from build123d import *

# Parameters (mm, degrees)
CORTAR_EXTRUIR1_START                       = 1
CROQUIS2_R                                  = 7.435198433
CORTAR_EXTRUIR1_DEPTH                       = 7
CHAFL_N1_SIZE                               = 0.1
DI_METRO_DE_TALADRO_1_0_1_1_D               = 1
DI_METRO_DE_TALADRO_1_0_1_1_DEPTH           = 0.2
DI_METRO_DE_TALADRO_1_0_1_1_TIP             = 0.30043031
DI_METRO_DE_TALADRO_1_0_1_1_ON_FACE_2_D     = 1
DI_METRO_DE_TALADRO_1_0_1_1_ON_FACE_2_DEPTH = 0.2
DI_METRO_DE_TALADRO_1_0_1_1_ON_FACE_2_TIP   = 0.30043031
DI_METRO_DE_TALADRO_1_0_1_1_ON_FACE_3_D     = 1
DI_METRO_DE_TALADRO_1_0_1_1_ON_FACE_3_DEPTH = 0.2
DI_METRO_DE_TALADRO_1_0_1_1_ON_FACE_3_TIP   = 0.30043031
DI_METRO_DE_TALADRO_1_0_1_1_ON_FACE_4_D     = 1
DI_METRO_DE_TALADRO_1_0_1_1_ON_FACE_4_DEPTH = 0.2
DI_METRO_DE_TALADRO_1_0_1_1_ON_FACE_4_TIP   = 0.30043031
DI_METRO_DE_TALADRO_1_0_1_1_ON_FACE_5_D     = 1
DI_METRO_DE_TALADRO_1_0_1_1_ON_FACE_5_DEPTH = 0.2
DI_METRO_DE_TALADRO_1_0_1_1_ON_FACE_5_TIP   = 0.30043031
DI_METRO_DE_TALADRO_1_0_1_1_ON_FACE_6_D     = 1
DI_METRO_DE_TALADRO_1_0_1_1_ON_FACE_6_DEPTH = 0.2
DI_METRO_DE_TALADRO_1_0_1_1_ON_FACE_6_TIP   = 0.30043031


with BuildPart() as part:
    # Croquis1 → Revolución1 (revolve)
    with BuildSketch(Plane.XY):
        with BuildLine():
            Line((0.5, 0), (0.575, 0))
            ThreePointArc((0.575, 0), (0.759699445, 0.045195667), (0.902660818, 0.170569425))
            Line((0.902660818, 0.170569425), (3.934160742, 4.5))
            Line((3.934160742, 4.5), (6.64058638, 4.5))
            Line((6.64058638, 4.5), (6.64058638, 8.36517638))
            Line((6.64058638, 8.36517638), (7.435198433, 9.5))
            Line((7.435198433, 9.5), (3, 9.5))
            Line((3, 9.5), (3, 19))
            Line((3, 19), (1.6, 19))
            Line((1.6, 19), (1.6, 3.570962807))
            Line((1.6, 3.570962807), (0.5, 2))
            Line((0.5, 2), (0.5, 0))
        make_face()
    revolve(axis=Axis((0, 0, 0), (0, 1, 0)))

    # Croquis2 → Cortar-Extruir1 (cut)
    with BuildSketch(Plane(origin=(0, 9.5, 0), x_dir=(1, 0, 0), z_dir=(0, 1, 0)).offset(CORTAR_EXTRUIR1_START)):
        Circle(CROQUIS2_R)
        Polygon((2.309401077, 4), (-2.309401077, 4), (-4.618802154, 0), (-2.309401077, -4), (2.309401077, -4), (4.618802154, 0), align=None, mode=Mode.SUBTRACT)
    extrude(amount=-CORTAR_EXTRUIR1_DEPTH, mode=Mode.SUBTRACT)

    # Chaflán1
    chafl_n1_edges = [part.edges().sort_by_distance(p)[0] for p in [
        (-1.6, 19, 0),
    ]]
    chamfer(chafl_n1_edges, length=CHAFL_N1_SIZE)

    # Diámetro de taladro Ø1.0 (1)1
    with Locations(Plane(origin=(0, 7, 4), x_dir=(1, 0, 0), z_dir=(0, 0, 1))):
        with Locations((0, 0)):
            Hole(DI_METRO_DE_TALADRO_1_0_1_1_D / 2, depth=DI_METRO_DE_TALADRO_1_0_1_1_DEPTH)
            with Locations((0, 0, -(DI_METRO_DE_TALADRO_1_0_1_1_DEPTH + DI_METRO_DE_TALADRO_1_0_1_1_TIP / 2))):  # 118° drill point
                Cone(0, DI_METRO_DE_TALADRO_1_0_1_1_D / 2, DI_METRO_DE_TALADRO_1_0_1_1_TIP, mode=Mode.SUBTRACT)

    # Diámetro de taladro Ø1.0 (1)1 on face 2
    with Locations(Plane(origin=(3.464101615, 7, 2), x_dir=(-0.500000175, 0, 0.866025303), z_dir=(0.866025303, 0, 0.500000175))):
        with Locations((0, 0)):
            Hole(DI_METRO_DE_TALADRO_1_0_1_1_ON_FACE_2_D / 2, depth=DI_METRO_DE_TALADRO_1_0_1_1_ON_FACE_2_DEPTH)
            with Locations((0, 0, -(DI_METRO_DE_TALADRO_1_0_1_1_ON_FACE_2_DEPTH + DI_METRO_DE_TALADRO_1_0_1_1_ON_FACE_2_TIP / 2))):  # 118° drill point
                Cone(0, DI_METRO_DE_TALADRO_1_0_1_1_ON_FACE_2_D / 2, DI_METRO_DE_TALADRO_1_0_1_1_ON_FACE_2_TIP, mode=Mode.SUBTRACT)

    # Diámetro de taladro Ø1.0 (1)1 on face 3
    with Locations(Plane(origin=(3.464101615, 7, -2), x_dir=(0.500000175, 0, 0.866025303), z_dir=(0.866025303, 0, -0.500000175))):
        with Locations((0, 0)):
            Hole(DI_METRO_DE_TALADRO_1_0_1_1_ON_FACE_3_D / 2, depth=DI_METRO_DE_TALADRO_1_0_1_1_ON_FACE_3_DEPTH)
            with Locations((0, 0, -(DI_METRO_DE_TALADRO_1_0_1_1_ON_FACE_3_DEPTH + DI_METRO_DE_TALADRO_1_0_1_1_ON_FACE_3_TIP / 2))):  # 118° drill point
                Cone(0, DI_METRO_DE_TALADRO_1_0_1_1_ON_FACE_3_D / 2, DI_METRO_DE_TALADRO_1_0_1_1_ON_FACE_3_TIP, mode=Mode.SUBTRACT)

    # Diámetro de taladro Ø1.0 (1)1 on face 4
    with Locations(Plane(origin=(0, 7, -4), x_dir=(-1, 0, 0), z_dir=(0, 0, -1))):
        with Locations((0, 0)):
            Hole(DI_METRO_DE_TALADRO_1_0_1_1_ON_FACE_4_D / 2, depth=DI_METRO_DE_TALADRO_1_0_1_1_ON_FACE_4_DEPTH)
            with Locations((0, 0, -(DI_METRO_DE_TALADRO_1_0_1_1_ON_FACE_4_DEPTH + DI_METRO_DE_TALADRO_1_0_1_1_ON_FACE_4_TIP / 2))):  # 118° drill point
                Cone(0, DI_METRO_DE_TALADRO_1_0_1_1_ON_FACE_4_D / 2, DI_METRO_DE_TALADRO_1_0_1_1_ON_FACE_4_TIP, mode=Mode.SUBTRACT)

    # Diámetro de taladro Ø1.0 (1)1 on face 5
    with Locations(Plane(origin=(-3.464101615, 7, -2), x_dir=(0.500000175, 0, -0.866025303), z_dir=(-0.866025303, 0, -0.500000175))):
        with Locations((0, 0)):
            Hole(DI_METRO_DE_TALADRO_1_0_1_1_ON_FACE_5_D / 2, depth=DI_METRO_DE_TALADRO_1_0_1_1_ON_FACE_5_DEPTH)
            with Locations((0, 0, -(DI_METRO_DE_TALADRO_1_0_1_1_ON_FACE_5_DEPTH + DI_METRO_DE_TALADRO_1_0_1_1_ON_FACE_5_TIP / 2))):  # 118° drill point
                Cone(0, DI_METRO_DE_TALADRO_1_0_1_1_ON_FACE_5_D / 2, DI_METRO_DE_TALADRO_1_0_1_1_ON_FACE_5_TIP, mode=Mode.SUBTRACT)

    # Diámetro de taladro Ø1.0 (1)1 on face 6
    with Locations(Plane(origin=(-3.464101615, 7, 2), x_dir=(-0.500000175, 0, -0.866025303), z_dir=(-0.866025303, 0, 0.500000175))):
        with Locations((0, 0)):
            Hole(DI_METRO_DE_TALADRO_1_0_1_1_ON_FACE_6_D / 2, depth=DI_METRO_DE_TALADRO_1_0_1_1_ON_FACE_6_DEPTH)
            with Locations((0, 0, -(DI_METRO_DE_TALADRO_1_0_1_1_ON_FACE_6_DEPTH + DI_METRO_DE_TALADRO_1_0_1_1_ON_FACE_6_TIP / 2))):  # 118° drill point
                Cone(0, DI_METRO_DE_TALADRO_1_0_1_1_ON_FACE_6_D / 2, DI_METRO_DE_TALADRO_1_0_1_1_ON_FACE_6_TIP, mode=Mode.SUBTRACT)


solid = part.part
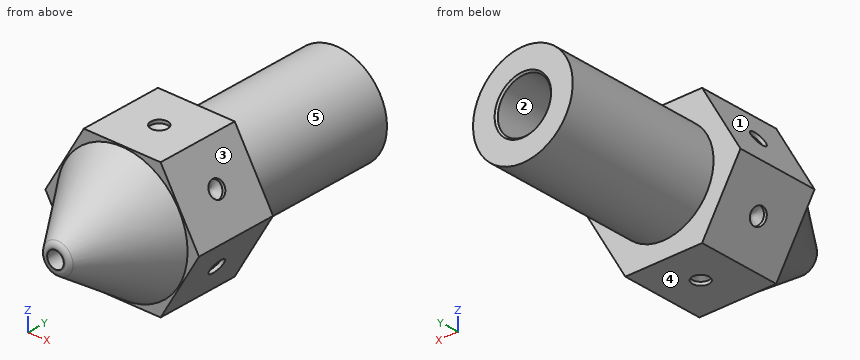
Geometry: final body of the model. Coordinates: model frame, mm. Face numbers are marked on the shaded views. A direction names the side the tool comes from. Coordinates: 2 decimals unless noted, no trailing zeros. Loops run counter-clockwise (first coordinate to the right, second up) from the corner with the lowest first, then second, coordinate; pieces in that order, holes last. Notation, with made-up numbers: M 43.5,-15 L 94.5,-15 A20 ccw 94.5,8 Z; hole C 11,-22.5 d3. An arc over 180 degrees is marked long. One line per item, written item: value. Start each with the question number.
1) Draft query along X for the marked faces 1, 2 and 3. Return one class per face: released by +X, released by -X, zero draft, split by the parting line, or undercut.
2) Cut plane B-B (x = 4.25). Return loops of the section in (y, z), then the cut area to 3 significant figures.
3) Cut plane A-A (y = 6.25). Return loops of the section in (x, z), then the cut area to 3 significant figures.
4) Reachability of the marked faces 4 and 5 from +Z, -Z, +X, -X, +Y, -Y: full face, straight path, thin tool, end or side. Return the list, or none.
5) Pin query (flat end, axial travel): P1, Ø3, axis at y = 13.5, z = 1.5, coming from the +X side; P2, Ø2, axis at y = 12.5, z = 3, coming from the -X side; P3, Ø4, axis at x = 1, y = 15.5, coming from the -Z side. Return the tip coordinate at first contact, or that it passes through.
6) Material intervals for L1, parallel to X at y = 7, z = 3.95; L2, parallel to Z at x = 0, y = 5.5; L3, parallel to Z at x = 0, y = 13.5, sorted ascending. Write a range as from..to.
7) Cut plane C-C (y = 13). Return loops of the section in (x, z), then the cut area to 3 significant figures.
Evaluation:
1. face 1: released by -X
1. face 2: undercut
1. face 3: released by +X
2. outline: M 4.5,-0.64 L 9.5,-0.64 L 9.5,0.64 L 4.5,0.64 Z
2. area: 6.39 mm^2
3. outline: M -4.62,0 L -2.31,-4 L 2.31,-4 L 4.62,0 L 2.31,4 L -2.31,4 Z; hole C 0,0 d3.2
3. area: 47.4 mm^2
4. face 4: -Z, +X, -X, +Y, -Y
4. face 5: +Y
5. P1: x = 3
5. P2: x = -2.24
5. P3: z = -3
6. L1: -2.34..-0.5, 0.5..2.34
6. L2: -4..-1.6, 1.6..4
6. L3: -3..-1.6, 1.6..3
7. outline: C 0,0 d6; hole C 0,0 d3.2
7. area: 20.2 mm^2
